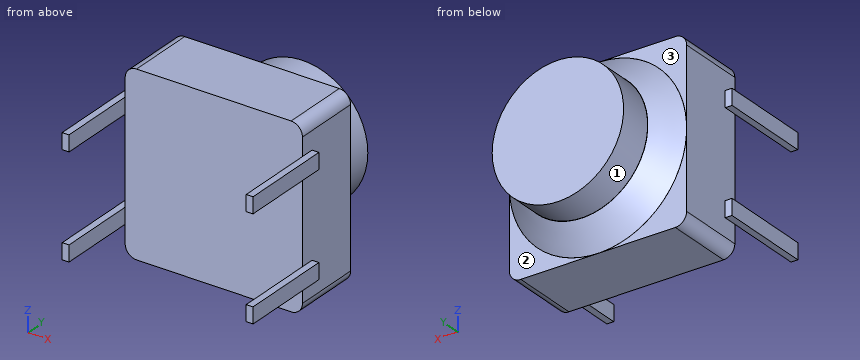
Solid Edge part; units mm, degrees
sketch "Sketch1" plane through (0, 0, 0) normal (0, -1, 0) x (1, 0, 0)
  line L0 (0, 0) -> (7.8, 0)
  line L1 (7.8, 0) -> (7.8, 7.8)
  line L2 (7.8, 7.8) -> (0, 7.8)
  line L3 (0, 7.8) -> (0, 0)
extrude "Protrusion1" add sketch "Sketch1" against normal blind 3
sketch "Sketch2" plane through (0, 0, 0) normal (0, -1, 0) x (1, 0, 0)
  circle A0 centre (3.9, 3.9) radius 3.9
extrude "Ajout_matière_3" add sketch "Sketch2" against normal blind 4
sketch "Sketch3" plane through (0, 0, 0) normal (0, -1, 0) x (1, 0, 0)
  circle A0 centre (3.9, 3.9) radius 2.8918
extrude "Ajout_matière_4" add sketch "Sketch3" against normal blind 5.5
chamfer "Chanfrein_1" distance 1 angle 45 1 edges at (0, 4, 3.9)
fillet "Congé_1" radius 0.5 4 edges at (7.8, 1.5, 7.8) (7.8, 1.5, 0) (0, 1.5, 0) (0, 1.5, 7.8)
sketch "Sketch4" plane through (3.9, 0, 3.9) normal (0, -1, 0) x (-1, 0, 0)
  line L0 (4.2, 1.9) -> (4.2, 2.6)
  line L1 (4.2, 2.6) -> (3.9, 2.6)
  line L2 (3.9, 2.6) -> (3.9, 1.9)
  line L3 (3.9, 1.9) -> (4.2, 1.9)
  line L4 (-4.2, 1.9) -> (-4.2, 2.6)
  line L5 (-4.2, 2.6) -> (-3.9, 2.6)
  line L6 (-3.9, 2.6) -> (-3.9, 1.9)
  line L7 (-3.9, 1.9) -> (-4.2, 1.9)
  line L8 (-4.2, -1.9) -> (-4.2, -2.6)
  line L9 (-4.2, -2.6) -> (-3.9, -2.6)
  line L10 (-3.9, -2.6) -> (-3.9, -1.9)
  line L11 (-3.9, -1.9) -> (-4.2, -1.9)
  line L12 (4.2, -1.9) -> (4.2, -2.6)
  line L13 (4.2, -2.6) -> (3.9, -2.6)
  line L14 (3.9, -2.6) -> (3.9, -1.9)
  line L15 (3.9, -1.9) -> (4.2, -1.9)
extrude "Ajout_matière_5" add sketch "Sketch4" against normal blind 0.6
sketch "Sketch5" plane through (3.9, 0, 3.9) normal (0, -1, 0) x (-1, 0, 0)
  line L0 (-4.2, 1.9) -> (-4.2, 2.6)
  line L1 (-4.2, 2.6) -> (-3.9, 2.6)
  line L2 (-3.9, 2.6) -> (-3.9, 1.9)
  line L3 (-3.9, 1.9) -> (-4.2, 1.9)
  line L4 (-4.2, -1.9) -> (-4.2, -2.6)
  line L5 (-4.2, -2.6) -> (-3.9, -2.6)
  line L6 (-3.9, -2.6) -> (-3.9, -1.9)
  line L7 (-3.9, -1.9) -> (-4.2, -1.9)
  line L8 (3.9, -2.6) -> (3.9, -1.9)
  line L9 (3.9, -1.9) -> (4.2, -1.9)
  line L10 (4.2, -1.9) -> (4.2, -2.6)
  line L11 (4.2, -2.6) -> (3.9, -2.6)
  line L12 (4.2, 1.9) -> (4.2, 2.6)
  line L13 (4.2, 2.6) -> (3.9, 2.6)
  line L14 (3.9, 2.6) -> (3.9, 1.9)
  line L15 (3.9, 1.9) -> (4.2, 1.9)
extrude "Ajout_matière_6" add sketch "Sketch5" along normal blind 3.5
CAD build for the part. Positions are in the model's coordinates, mm. Face numbers are marked on the shaded views. A direction names the side the tool comes from. Coordinates: 2 decimals unless noted, no trailing zeros. Order: outer loops, then holes, each group sorted by start corner. A loop starts at its lowest first (then second) coordinate and runs counter-clockwise, first axis right, second up. Notation, with made-up numbers: M 53,70.5 L 110,70.5 A22 cw 110,77.5 Z; hole C 31,55 d6. An arc over 180 degrees is marked long. Answer as CSV lines item,"result".
1) Cut at B-B (y = 2.25). List the corners of the cut face in (x, z).
Verdict:
outline,"M 0,0.5 A0.5 ccw 0.5,0 L 7.3,0 A0.5 ccw 7.8,0.5 L 7.8,7.3 A0.5 ccw 7.3,7.8 L 0.5,7.8 A0.5 ccw 0,7.3 Z"
2) Drill centre lines: L1, parallel to X at y = 2.5, z = 3; L2, parallel to Y at x = 3.5, z = 2.25; L3, parallel to Y at x = 7.5, z = 6.75. Where is each one in solid material? Low to high. Write a range as from..to.
Verdict:
L1,"0..7.8"
L2,"0..5.5"
L3,"0..3"
3) Flat gauge pins, fed straight in: P1, Ø1.2, axis at x = 6.5, z = 1.5, coming from the +Y side; P2, Ø1, axis at y = 0.5, z = 5, coming from the +X side; P3, Ø2.5, axis at y = 2, z = 4, coming from the -X side. Where does each tip first touch, or does it go through?
Verdict:
P1,"y = 3.96"
P2,"x = 7.8"
P3,"x = 0"
4) 3-axis set-ups, long thin cutter, end or side, ignore diameter. For the marked faces 1, 2 and 3: which of +Z, -Z, +X, -X, +Y, -Y reach the whole face in a straight line?
Verdict:
face 1,"+Y"
face 2,"-Z, +X, +Y"
face 3,"+Z, -X, +Y"
5) Cut at A-A (y = -1.75). List the corners of the cut face in (x, z).
Verdict:
outline,"M -0.3,1.3 L 0,1.3 L 0,2 L -0.3,2 Z; M -0.3,5.8 L 0,5.8 L 0,6.5 L -0.3,6.5 Z; M 7.8,1.3 L 8.1,1.3 L 8.1,2 L 7.8,2 Z; M 7.8,5.8 L 8.1,5.8 L 8.1,6.5 L 7.8,6.5 Z"
6) Cut at C-C (y = 5.25). List the corners of the cut face in (x, z).
Verdict:
outline,"C 3.9,3.9 d5.78"
